```python
from build123d import *

# Parameters (mm, degrees)
SKETCH1_R           = 4.7625
SKETCH1_R_2         = 2.032
BOSS_EXTRUDE1_DEPTH = 3.175
BOSS_EXTRUDE2_START = -3.175
SKETCH2_R           = 6
BOSS_EXTRUDE2_DEPTH = 3.175


with BuildPart() as part:
    # Sketch1 → Boss-Extrude1 (new body)
    with BuildSketch(Plane.XY):
        with BuildLine():
            Line((43.65625, -13.0556), (-16.66875, -13.0556))
            ThreePointArc((-16.66875, -13.0556), (-20.036346045, -11.660696045), (-21.43125, -8.2931))
            Line((-21.43125, -8.2931), (-21.43125, 8.2931))
            ThreePointArc((-21.43125, 8.2931), (-20.036346045, 11.660696045), (-16.66875, 13.0556))
            Line((-16.66875, 13.0556), (43.65625, 13.0556))
            ThreePointArc((43.65625, 13.0556), (47.023846045, 11.660696045), (48.41875, 8.2931))
            Line((48.41875, 8.2931), (48.41875, -8.2931))
            ThreePointArc((48.41875, -8.2931), (47.023846045, -11.660696045), (43.65625, -13.0556))
        make_face()
        with Locations((26.9875, 0)):
            Circle(SKETCH1_R, mode=Mode.SUBTRACT)
        with Locations((-16.66875, 8.2931)):
            Circle(SKETCH1_R_2, mode=Mode.SUBTRACT)
        with Locations((43.65625, 8.2931)):
            Circle(SKETCH1_R_2, mode=Mode.SUBTRACT)
        with Locations((-16.66875, -8.2931)):
            Circle(SKETCH1_R_2, mode=Mode.SUBTRACT)
        with Locations((43.65625, -8.2931)):
            Circle(SKETCH1_R_2, mode=Mode.SUBTRACT)
        with Locations((-1.27, 0)):
            Circle(SKETCH1_R_2, mode=Mode.SUBTRACT)
    extrude(amount=BOSS_EXTRUDE1_DEPTH)

    # Sketch2 → Boss-Extrude2 (add)
    with BuildSketch(Plane.XY.offset(3.175).offset(BOSS_EXTRUDE2_START)):
        with BuildLine():
            Line((22.98118695, -31.924816254), (-18.671906525, -12.613837227))
            ThreePointArc((-18.671906525, -12.613837227), (-17.694394969, -12.943848181), (-16.66875, -13.0556))
            Line((-16.66875, -13.0556), (43.65625, -13.0556))
            ThreePointArc((43.65625, -13.0556), (45.826918249, -12.53215716), (47.520433425, -11.076891067))
            Line((47.520433425, -11.076891067), (34.71586685, -28.850923935))
            ThreePointArc((34.71586685, -28.850923935), (29.401133075, -32.49746142), (22.98118695, -31.924816254))
        make_face()
        with Locations((26.9875, -23.2833418)):
            Circle(SKETCH2_R, mode=Mode.SUBTRACT)
    extrude(amount=BOSS_EXTRUDE2_DEPTH)


solid = part.part
```
For this review, take the finished solid that the model builds, in its own axes (mm). Coordinates: 2 decimals unless noted, no trailing zeros. Loops run counter-clockwise (first coordinate to the right, second up) from the corner with the lowest first, then second, coordinate; pieces in that order, holes last.
1. Add section D-D, the plane y = -24.5. Give the boundary of the cut face in (x, z) (3 decimals).
2. Mouldability with a two-part tool opening along X and no side actions: class faces 1 (the cylindrical face through (46.987, 11.698, 1.565)), 2 (the flat face through (14, -4, 0)), 3 (the cylindrical face through (-18.7, -8.2, 1.6)) as +X half, -X half, draft (parallel to the pull), parting line (faces both ways), or undercut.
3. Add section A-A, the plane y = 0. Give the boundary of the cut face in (x, z) (3 decimals).
4. Add section C-C, the plane z = 1.5. Count the separate pieces of the cut face and the enclosed holes in it, then the cut area to 3 significant figures.
5. For line 1 (Y direction, x = 23.5, z = 2.7); line 2 (Y direction, x = -17, z = 2.55); line 3 (Y direction, x = -1, z = 1.35), list the stretches that pass through material, from the lowest coordinate up.
6. Insertion check: P1, Ø15.5, axis at x = 26.99, y = -23.28, coming from the -Z side; P2, Ø1, axis at x = 38.5, z = 2, coming from the -Y side. Each pin has a flat end and moves straight along its axis. Give the tip position at first contact, or say it passes through.
7. Add section B-B, the plane x = 30. Give the boundary of the cut face in (y, z) (3 decimals), then the cut area to 3 significant figures.
Result:
1. outline: (6.966, 0) - (21.112, 0) - (21.112, 3.175) - (6.966, 3.175) - close; (32.863, 0) - (37.85, 0) - (37.85, 3.175) - (32.863, 3.175) - close
2. face 1: +X half
2. face 2: draft
2. face 3: undercut
3. outline: (-21.431, 0) - (-3.302, 0) - (-3.302, 3.175) - (-21.431, 3.175) - close; (0.762, 0) - (22.225, 0) - (22.225, 3.175) - (0.762, 3.175) - close; (31.75, 0) - (48.419, 0) - (48.419, 3.175) - (31.75, 3.175) - close
4. separate pieces: 1
4. enclosed holes: 7
4. area: 2,250 mm2
5. line 1: y = -32.15 to -28.17, -18.4 to -3.24, 3.24 to 13.06
5. line 2: y = -13.39 to -10.3, -6.29 to 6.29, 10.3 to 13.04
5. line 3: y = -20.81 to -2.01, 2.01 to 13.06
6. P1: stops at z = 0
6. P2: stops at y = -24.29
7. outline: (-32.319, 0) - (-28.472, 0) - (-28.472, 3.175) - (-32.319, 3.175) - close; (-18.094, 0) - (-3.689, 0) - (-3.689, 3.175) - (-18.094, 3.175) - close; (3.689, 0) - (13.056, 0) - (13.056, 3.175) - (3.689, 3.175) - close
7. area: 87.7 mm2
